Verification items for the finished model (mm, model axes). A direction names the side the tool comes from. Round coordinates to 2 decimals unless told otherwise and drop trailing zeros. Loops run counter-clockwise (first coordinate to the right, second up) from the corner with the lowest first, then second, coordinate; pieces in that order, holes last. Notation, with made-up numbers: M -38.75,42.5 L 12.25,42.5 A24 ccw 12.25,64.5 Z; hole C 1.25,26.25 d9. An arc over 180 degrees is marked long. One line per item, written item: value.
from build123d import *

# Parameters (mm, degrees)
CROQUIS5_R              = 24.5
SALIENTE_EXTRUIR3_DEPTH = 3.2
SALIENTE_EXTRUIR4_DEPTH = 3.2
CROQUIS7_R              = 50
SALIENTE_EXTRUIR5_DEPTH = 3.5
CROQUIS8_W              = 5
CROQUIS8_H              = 5
CORTAR_EXTRUIR3_DEPTH   = 3
CROQUIS9_R              = 3.535533906
CORTAR_EXTRUIR4_DEPTH   = 2.5


with BuildPart() as part:
    # Croquis5 → Saliente-Extruir3 (new body)
    with BuildSketch(Plane(origin=(0, 0, 0), x_dir=(1, 0, 0), z_dir=(0, 1, 0))):
        with Locations(Location((0, 0, 0), (0, 0, 270))):
            Circle(CROQUIS5_R)
    extrude(amount=SALIENTE_EXTRUIR3_DEPTH)

    # Croquis6 → Saliente-Extruir4 (add)
    with BuildSketch(Plane.XZ):
        with BuildLine():
            Line((33.5, 4.8), (-33.5, 4.8))
            ThreePointArc((-33.5, 4.8), (-34.207106781, 4.507106781), (-34.5, 3.8))
            Line((-34.5, 3.8), (-34.5, -3.8))
            ThreePointArc((-34.5, -3.8), (-34.207106781, -4.507106781), (-33.5, -4.8))
            Line((-33.5, -4.8), (33.5, -4.8))
            ThreePointArc((33.5, -4.8), (34.207106781, -4.507106781), (34.5, -3.8))
            Line((34.5, -3.8), (34.5, 3.8))
            ThreePointArc((34.5, 3.8), (34.207106781, 4.507106781), (33.5, 4.8))
        make_face()
        with BuildLine():
            Line((3.8, -34.5), (-3.8, -34.5))
            ThreePointArc((-3.8, -34.5), (-4.507106781, -34.207106781), (-4.8, -33.5))
            Line((-4.8, -33.5), (-4.8, 33.5))
            ThreePointArc((-4.8, 33.5), (-4.507106781, 34.207106781), (-3.8, 34.5))
            Line((-3.8, 34.5), (3.8, 34.5))
            ThreePointArc((3.8, 34.5), (4.507106781, 34.207106781), (4.8, 33.5))
            Line((4.8, 33.5), (4.8, -33.5))
            ThreePointArc((4.8, -33.5), (4.507106781, -34.207106781), (3.8, -34.5))
        make_face()
    extrude(amount=-SALIENTE_EXTRUIR4_DEPTH)

    # Croquis7 → Saliente-Extruir5 (add)
    with BuildSketch(Plane.XZ):
        with Locations(Location((0, 0, 0), (0, 0, 270))):
            Circle(CROQUIS7_R)
    extrude(amount=SALIENTE_EXTRUIR5_DEPTH)

    # Croquis8 → Cortar-Extruir3 (cut)
    with BuildSketch(Plane.XZ.offset(3.5)):
        with BuildLine():
            Line((-2.5, -25), (2.5, -25))
            Line((2.5, -25), (2.5, -19.843134833))
            ThreePointArc((2.5, -19.843134833), (0, -20), (-2.5, -19.843134833))
            Line((-2.5, -19.843134833), (-2.5, -25))
        make_face()
        with BuildLine():
            ThreePointArc((-2.5, -19.843134833), (0, -20), (2.5, -19.843134833))
            Line((2.5, -19.843134833), (2.5, -14.790199458))
            ThreePointArc((2.5, -14.790199458), (0, -15), (-2.5, -14.790199458))
            Line((-2.5, -14.790199458), (-2.5, -19.843134833))
        make_face()
        with BuildLine():
            ThreePointArc((2.5, 19.843134833), (0, 20), (-2.5, 19.843134833))
            Line((-2.5, 19.843134833), (-2.5, 14.790199458))
            ThreePointArc((-2.5, 14.790199458), (0, 15), (2.5, 14.790199458))
            Line((2.5, 14.790199458), (2.5, 19.843134833))
        make_face()
        with BuildLine():
            ThreePointArc((-2.5, -14.790199458), (0, -15), (2.5, -14.790199458))
            Line((2.5, -14.790199458), (2.5, -2.5))
            Line((2.5, -2.5), (-2.5, -2.5))
            Line((-2.5, -2.5), (-2.5, -14.790199458))
        make_face()
        Rectangle(CROQUIS8_W, CROQUIS8_H)
        with BuildLine():
            Line((-2.5, 2.5), (2.5, 2.5))
            Line((2.5, 2.5), (2.5, 14.790199458))
            ThreePointArc((2.5, 14.790199458), (0, 15), (-2.5, 14.790199458))
            Line((-2.5, 14.790199458), (-2.5, 2.5))
        make_face()
        with BuildLine():
            Line((-2.5, 25), (-2.5, 19.843134833))
            ThreePointArc((-2.5, 19.843134833), (0, 20), (2.5, 19.843134833))
            Line((2.5, 19.843134833), (2.5, 25))
            Line((2.5, 25), (-2.5, 25))
        make_face()
        with BuildLine():
            Line((2.5, 2.5), (2.5, -2.5))
            Line((2.5, -2.5), (14.790199458, -2.5))
            ThreePointArc((14.790199458, -2.5), (14.947457842, -1.254393904), (15, 0))
            ThreePointArc((15, 0), (14.947457842, 1.254393904), (14.790199458, 2.5))
            Line((14.790199458, 2.5), (2.5, 2.5))
        make_face()
        with BuildLine():
            Line((14.790199458, -2.5), (19.843134833, -2.5))
            ThreePointArc((19.843134833, -2.5), (19.960745185, -1.252458251), (20, 0))
            ThreePointArc((20, 0), (19.960745185, 1.252458251), (19.843134833, 2.5))
            Line((19.843134833, 2.5), (14.790199458, 2.5))
            ThreePointArc((14.790199458, 2.5), (14.947457842, 1.254393904), (15, 0))
            ThreePointArc((15, 0), (14.947457842, -1.254393904), (14.790199458, -2.5))
        make_face()
        with BuildLine():
            ThreePointArc((-19.843134833, 2.5), (-20, 0), (-19.843134833, -2.5))
            Line((-19.843134833, -2.5), (-14.790199458, -2.5))
            ThreePointArc((-14.790199458, -2.5), (-15, 0), (-14.790199458, 2.5))
            Line((-14.790199458, 2.5), (-19.843134833, 2.5))
        make_face()
        with BuildLine():
            ThreePointArc((20, 0), (19.960745185, -1.252458251), (19.843134833, -2.5))
            Line((19.843134833, -2.5), (25, -2.5))
            Line((25, -2.5), (25, 2.5))
            Line((25, 2.5), (19.843134833, 2.5))
            ThreePointArc((19.843134833, 2.5), (19.960745185, 1.252458251), (20, 0))
        make_face()
        with BuildLine():
            Line((-14.790199458, -2.5), (-2.5, -2.5))
            Line((-2.5, -2.5), (-2.5, 2.5))
            Line((-2.5, 2.5), (-14.790199458, 2.5))
            ThreePointArc((-14.790199458, 2.5), (-15, 0), (-14.790199458, -2.5))
        make_face()
        with BuildLine():
            Line((-25, -2.5), (-19.843134833, -2.5))
            ThreePointArc((-19.843134833, -2.5), (-20, 0), (-19.843134833, 2.5))
            Line((-19.843134833, 2.5), (-25, 2.5))
            Line((-25, 2.5), (-25, -2.5))
        make_face()
        with BuildLine():
            ThreePointArc((-2.5, 19.843134833), (-14.142135624, 14.142135624), (-19.843134833, 2.5))
            Line((-19.843134833, 2.5), (-14.790199458, 2.5))
            ThreePointArc((-14.790199458, 2.5), (-10.606601718, 10.606601718), (-2.5, 14.790199458))
            Line((-2.5, 14.790199458), (-2.5, 19.843134833))
        make_face()
        with BuildLine():
            Line((14.790199458, 2.5), (19.843134833, 2.5))
            ThreePointArc((19.843134833, 2.5), (14.142135624, 14.142135624), (2.5, 19.843134833))
            Line((2.5, 19.843134833), (2.5, 14.790199458))
            ThreePointArc((2.5, 14.790199458), (10.606601718, 10.606601718), (14.790199458, 2.5))
        make_face()
        with BuildLine():
            Line((2.5, -14.790199458), (2.5, -19.843134833))
            ThreePointArc((2.5, -19.843134833), (14.142135624, -14.142135624), (19.843134833, -2.5))
            Line((19.843134833, -2.5), (14.790199458, -2.5))
            ThreePointArc((14.790199458, -2.5), (10.606601718, -10.606601718), (2.5, -14.790199458))
        make_face()
        with BuildLine():
            ThreePointArc((-19.843134833, -2.5), (-14.142135624, -14.142135624), (-2.5, -19.843134833))
            Line((-2.5, -19.843134833), (-2.5, -14.790199458))
            ThreePointArc((-2.5, -14.790199458), (-10.606601718, -10.606601718), (-14.790199458, -2.5))
            Line((-14.790199458, -2.5), (-19.843134833, -2.5))
        make_face()
    extrude(amount=-CORTAR_EXTRUIR3_DEPTH, mode=Mode.SUBTRACT)

    # Croquis9 → Cortar-Extruir4 (cut)
    with BuildSketch(Plane.XZ.offset(0.5)):
        with Locations(Location((0, 0, 0), (0, 0, 270))):
            Circle(CROQUIS9_R)
    extrude(amount=-CORTAR_EXTRUIR4_DEPTH, mode=Mode.SUBTRACT)


solid = part.part
(1) Sectioned sample at B-B on x = 0. Enter the section's corners in (y, z), and give its area (3 significant figures).
Completed:
outline: M -3.5,-50 L 0,-50 L 0,-34.5 L 3.2,-34.5 L 3.2,34.5 L 0,34.5 L 0,50 L -3.5,50 L -3.5,25 L -0.5,25 L -0.5,3.54 L 2,3.54 L 2,-3.54 L -0.5,-3.54 L -0.5,-25 L -3.5,-25 Z
area: 403 mm^2
(2) Sectioned sample at C-C on z = -6. Enter the section's corners in (x, y).
Completed:
outline: M -49.64,-3.5 L -19.08,-3.5 L -19.08,-0.5 L -13.75,-0.5 L -13.75,-3.5 L -2.5,-3.5 L -2.5,-0.5 L 2.5,-0.5 L 2.5,-3.5 L 13.75,-3.5 L 13.75,-0.5 L 19.08,-0.5 L 19.08,-3.5 L 49.64,-3.5 L 49.64,0 L 23.75,0 L 23.75,3.2 L -23.75,3.2 L -23.75,0 L -49.64,0 Z
(3) Tool access check on faces 1 (the face through (-22, -3.5, -10)), 2 (the face through (-25, -2, 0)). Record the directions out of +Z, -Z, +X, -X, +Y, -Y that give a thin tool (end or side, any length) a straight path to the whole face; none if there is none.
Completed:
face 1: +Z, -Z, +X, -X, -Y
face 2: -Y
(4) Mould release check, pull along X, two halves, no side actions. Record for faces 3 (the face through (-4.8, 2, -29)), 4 (the face through (12, 0, -22)), 5 (the face through (22, -2, -2.5)), 6 (the face through (4.8, 2, -29)): +X half, -X half, draft (parallel to the pull), parting line (faces both ways), or undercut.
Completed:
face 3: -X half
face 4: draft
face 5: undercut
face 6: +X half
(5) Depth check by flat-ended pin: pin 1 Ø2 at (x, y) = (35, -0.5) entering from -Z; pin 2 Ø3 at (x, y) = (3, -2.5) entering from -Z; pin 3 Ø2.5 at (y, z) = (2, -29.5) entering from +X. Enter the tip coordinate at first touch or a pass-through.
Completed:
pin 1: stops at z = -36.66
pin 2: stops at z = -49.98
pin 3: stops at x = 4.8
(6) Thickness scan on L1, parallel to Z at x = 0, y = 0.8; L2, parallel to X at y = -0.75, z = -9.5. Record the ranges inside material, lowest first. Write a range as from..to.
Completed:
L1: z = -34.5..-3.54, 3.54..34.5
L2: x = -49.09..-17.6, -11.61..-2.5, 2.5..11.61, 17.6..49.09
(7) Sectioned sample at A-A on y = -1.75. Count the separate pieces of the cut face and the enclosed holes in it, and give its area (3 significant figures).
Completed:
separate pieces: 5
enclosed holes: 1
area: 6,930 mm^2
(8) Sectioned sample at D-D on x = 21.5. Enter the section's corners in (y, z).
Completed:
outline: M -3.5,-45.14 L 0,-45.14 L 0,-11.75 L 3.2,-11.75 L 3.2,11.75 L 0,11.75 L 0,45.14 L -3.5,45.14 L -3.5,2.5 L -0.5,2.5 L -0.5,-2.5 L -3.5,-2.5 Z
